```python
from build123d import *

# Parameters (mm, degrees)
SKETCH1_R           = 12.5
SKETCH1_R_2         = 10.5
BOSS_EXTRUDE1_DEPTH = 20
BOSS_EXTRUDE2_DEPTH = 1
CIRPATTERN1_COUNT   = 3


with BuildPart() as part:
    # Sketch1 → Boss-Extrude1 (new body)
    with BuildSketch(Plane(origin=(0, 0, 0), x_dir=(1, 0, 0), z_dir=(0, 1, 0))):
        Circle(SKETCH1_R)
        Circle(SKETCH1_R_2, mode=Mode.SUBTRACT)
    extrude(amount=BOSS_EXTRUDE1_DEPTH)

    # Sketch4 → Boss-Extrude2 (add)
    with BuildSketch(Plane(origin=(0, 0, 0), x_dir=(0, 0, 1), z_dir=(0.707106781, 0.707106781, 0))):
        with BuildLine():
            Line((-9.363412571, -8.137222405), (0, -1.322062821))
            Line((0, -1.322062821), (9.559751039, -8.008067831))
            ThreePointArc((9.559751039, -8.008067831), (0.151357729, -15.865590891), (-9.363412571, -8.137222405))
        make_face()
    boss_extrude2 = extrude(amount=-BOSS_EXTRUDE2_DEPTH)

    # CirPattern1: Boss-Extrude2 ×3 about axis
    cirpattern1_axis = Axis((0, 0, 0), (0, 1, 0))
    for i in range(1, CIRPATTERN1_COUNT):
        add(boss_extrude2.rotate(cirpattern1_axis, i * 360 / CIRPATTERN1_COUNT))


solid = part.part
```
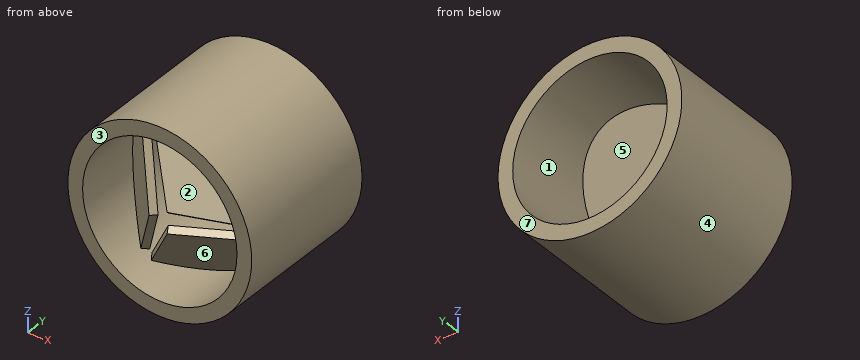
Input: part model. Units: mm. Frame: model coordinates. Face numbers are marked on the shaded views. A direction names the side the tool comes from. Round coordinates to 2 decimals unless told otherwise and drop trailing zeros. Loops run counter-clockwise (first coordinate to the right, second up) from the corner with the lowest first, then second, coordinate; pieces in that order, holes last.
1) Section query B-B on x = -3.75. Return the cut outline in (y, z).
Ans:
outline: (0, -11.92) - (20, -11.92) - (20, -9.81) - (6.62, -9.81) - (4.31, -7.14) - (3.88, -8.28) - (5.2, -9.81) - (0, -9.81) - close; (0, 9.81) - (5.2, 9.81) - (4.09, 8.52) - (4.5, 7.36) - (6.62, 9.81) - (20, 9.81) - (20, 11.92) - (0, 11.92) - close; (2.34, -4.1) - (3.75, -5.47) - (3.75, 5.69) - (2.34, 4.26) - close
2) Section query A-A on z = 5.5. Return the cut outline in (x, y).
Ans:
outline: (-11.22, 0) - (-8.94, 0) - (-8.94, 7.53) - (-4.36, 2.95) - (-3.65, 3.65) - (-8.94, 8.94) - (-8.94, 20) - (-11.22, 20) - close; (-2.55, 3.49) - (-1.8, 2.45) - (8.94, 7.82) - (8.94, 0) - (11.22, 0) - (11.22, 20) - (8.94, 20) - (8.94, 9.24) - close
3) Set-up query: the marked faces 1, 2 and 3. Return all of +Z, -Z, +X, -X, +Y, -Y with unobstructed straight access to the full face (end or side cutting, diameter ignored); none if empty.
Ans:
face 1: none
face 2: -Y
face 3: +Z, -Z, +X, -X, -Y
4) Section query C-C on x = 0. Return the cut outline in (y, z).
Ans:
outline: (0, -12.5) - (20, -12.5) - (20, -10.5) - (9.09, -10.5) - (1.31, -1.51) - (0.88, -2.65) - (7.68, -10.5) - (0, -10.5) - close; (0, 10.5) - (7.68, 10.5) - (0.92, 2.7) - (1.33, 1.54) - (9.09, 10.5) - (20, 10.5) - (20, 12.5) - (0, 12.5) - close
5) Material intervals for line 1 (X direction, y = 10.5, z = 0); line 2 (X direction, y = 6.5, z = 4.5); line 3 (X direction, y = 8.75, z = -8.25), sorted ascending.
Ans:
line 1: x = -12.5 to -10.5, 10.5 to 12.5
line 2: x = -11.66 to -9.49, -7.91 to -6.5, 5.21 to 8.03, 9.49 to 11.66
line 3: x = -9.39 to -6.5, 3.21 to 6.04, 6.5 to 9.39
6) Pin query (flat end, axial travel): pin 1 (12 mm diameter, centred on x = -0.5, z = 4, fed in from +Y); pin 2 (1 mm diameter, centred on y = 10, z = -6, fed in from +X) (3 decimals); pin 3 (12 mm diameter, centred on x = -1.5, z = -2.5, fed in from -Y). Return the tip coordinate at first contact, or that it passes through.
Ans:
pin 1: stops at y = 9.21
pin 2: stops at x = 11.225
pin 3: stops at y = 0.23
7) Section query D-D on y = 7. Return the cut outline in (x, z).
Ans:
outline: circle Ø25 at (0, 0); hole (-8.41, -6.28) - (-8.41, 6.28) arc R10.5 ccw to start; hole (-7, -7.83) arc R10.5 ccw to (-3.28, -9.98) - (10.28, -2.15) arc R10.5 ccw to (10.28, 2.15) - (-3.28, 9.98) arc R10.5 ccw to (-7, 7.83) - close; hole (-1.23, -10.43) arc R10.5 ccw to (9.65, -4.15) - close; hole (-1.23, 10.43) - (9.65, 4.15) arc R10.5 ccw to start
8) Pull-direction query (X, two-part tool) for the marked faces 4, 5, 6 and 7; classes: released by +X, released by -X, zero draft, split by the parting line, or undercut.
Ans:
face 4: split by the parting line
face 5: undercut
face 6: undercut
face 7: zero draft
